from build123d import *

# Parameters (mm, degrees)
SKETCH_1_W          = 40
SKETCH_1_H          = 25
EXTRUDE_1_DEPTH     = 3
SKETCH_2_R          = 10.9
EXTRUDE_2_DEPTH     = 5
SKETCH_3_R          = 4
CUT_EXTRUDE_1_DEPTH = 25.904818811
CUT_EXTRUDE_2_DEPTH = 3.6
SKETCH_5_R          = 0.5
CUT_EXTRUDE_3_DEPTH = 4
FILLET_1_R          = 5
FILLET_2_R          = 5
FILLET_3_R          = 5
FILLET_4_R          = 5
SKETCH_6_R          = 7
SKETCH_6_R_2        = 3
EXTRUDE_3_DEPTH     = 10
SKETCH_7_R          = 4
SKETCH_7_R_2        = 2
EXTRUDE_4_DEPTH     = 3


with BuildPart() as part:
    # 草图1 → 凸台-拉伸1 (new body)
    with BuildSketch(Plane(origin=(0, 0, 0), x_dir=(1, 0, 0), z_dir=(0, 1, 0))):
        Rectangle(SKETCH_1_W, SKETCH_1_H)
    extrude(amount=EXTRUDE_1_DEPTH)

    # 草图2 → 凸台-拉伸2 (add)
    with BuildSketch(Plane(origin=(0, 3, 0), x_dir=(1, 0, 0), z_dir=(0, 1, 0))):
        with Locations(Location((0, 0, 0), (0, 0, 270))):
            Circle(SKETCH_2_R)
    extrude(amount=EXTRUDE_2_DEPTH)

    # 草图3 → 切除-拉伸1 (cut, through all)
    with BuildSketch(Plane.XZ):
        with Locations(Location((0, 0, 0), (0, 0, 270))):
            Circle(SKETCH_3_R)
    extrude(amount=-CUT_EXTRUDE_1_DEPTH, mode=Mode.SUBTRACT)

    # 草图4 → 切除-拉伸2 (cut)
    with BuildSketch(Plane(origin=(0, 8, 0), x_dir=(1, 0, 0), z_dir=(0, 1, 0))):
        Polygon((3.674809939, -1.579801226), (2.341337155, -12.320336373), (-2.341337155, -12.320336373), (-3.674809939, -1.579801226), align=None)
        Polygon((-3.674809939, 1.579801226), (-2.341337155, 12.320336373), (2.341337155, 12.320336373), (3.674809939, 1.579801226), align=None)
    extrude(amount=-CUT_EXTRUDE_2_DEPTH, mode=Mode.SUBTRACT)

    # 草图5 → 切除-拉伸3 (cut)
    with BuildSketch(Plane(origin=(0, 4.4, 0), x_dir=(1, 0, 0), z_dir=(0, 1, 0))):
        with Locations(Location((0, -6.5, 0), (0, 0, 270))):
            Circle(SKETCH_5_R)
        with Locations(Location((0, 6.5, 0), (0, 0, 270))):
            Circle(SKETCH_5_R)
    extrude(amount=-CUT_EXTRUDE_3_DEPTH, mode=Mode.SUBTRACT)

    # 圆角1
    fillet_1_edges = [part.edges().sort_by_distance(p)[0] for p in [
        (20, 1.5, 12.5),
    ]]
    fillet(fillet_1_edges, radius=FILLET_1_R)

    # 圆角2
    fillet_2_edges = [part.edges().sort_by_distance(p)[0] for p in [
        (-20, 1.5, 12.5),
    ]]
    fillet(fillet_2_edges, radius=FILLET_2_R)

    # 圆角3
    fillet_3_edges = [part.edges().sort_by_distance(p)[0] for p in [
        (-20, 1.5, -12.5),
    ]]
    fillet(fillet_3_edges, radius=FILLET_3_R)

    # 圆角4
    fillet_4_edges = [part.edges().sort_by_distance(p)[0] for p in [
        (20, 1.5, -12.5),
    ]]
    fillet(fillet_4_edges, radius=FILLET_4_R)

    # 草图6 → 凸台-拉伸3 (add)
    with BuildSketch(Plane(origin=(0, 0, 0), x_dir=(-1, 0, 0), z_dir=(0, -1, 0))):
        with Locations(Location((0, 0, 0), (0, 0, 270))):
            Circle(SKETCH_6_R)
        with Locations(Location((0, 0, 0), (0, 0, 90))):
            Circle(SKETCH_6_R_2, mode=Mode.SUBTRACT)
    extrude(amount=EXTRUDE_3_DEPTH)

    # 草图7 → 凸台-拉伸4 (add)
    with BuildSketch(Plane(origin=(0, 0, 0), x_dir=(1, 0, 0), z_dir=(0, 1, 0))):
        with Locations(Location((0, 0, 0), (0, 0, 156.73712516))):
            Circle(SKETCH_7_R)
        with Locations(Location((0, 0, 0), (0, 0, 270))):
            Circle(SKETCH_7_R_2, mode=Mode.SUBTRACT)
    extrude(amount=EXTRUDE_4_DEPTH)


solid = part.part
The listing builds one solid part. Answer for the finished solid, in the listing's coordinates (mm). A direction names the side the tool comes from. Give positions to 0.01 mm unless a question says otherwise; leave off trailing zeros. Loops run counter-clockwise (first coordinate to the right, second up) from the corner with the lowest first, then second, coordinate; pieces in that order, holes last.
Item 1: Each of these flat-tipped pins is pushed along its axis until it touches: pin 1 Ø0.8 at (x, z) = (0, 6.5) entering from +Y; pin 2 Ø4 at (x, z) = (-1, 1) entering from +Y; pin 3 Ø1.5 at (x, z) = (7, -8) entering from -Y. Where does it stop, or does it pass through?
Derived:
pin 1: stops at y = 0.4
pin 2: stops at y = 3
pin 3: stops at y = 0
Item 2: A cutting plane is placed at D-D (z = 9.25). Give the vertices of the cut face in (x, y), then the cut area to 3 significant figures.
Derived:
outline: (-19.68, 0) - (19.68, 0) - (19.68, 3) - (5.77, 3) - (5.77, 8) - (2.72, 8) - (2.72, 4.4) - (-2.72, 4.4) - (-2.72, 8) - (-5.77, 8) - (-5.77, 3) - (-19.68, 3) - close
area: 156 mm2
Item 3: A cutting plane is placed at C-C (y = 2). Give the vertices of the cut face in (x, z).
Derived:
outline: (-20, -7.5) arc R5 ccw to (-15, -12.5) - (15, -12.5) arc R5 ccw to (20, -7.5) - (20, 7.5) arc R5 ccw to (15, 12.5) - (-15, 12.5) arc R5 ccw to (-20, 7.5) - close; hole circle Ø4 at (0, 0); hole circle Ø1 at (0, -6.5); hole circle Ø1 at (0, 6.5)
Item 4: A cutting plane is placed at A-A (z = 0). Give the vertices of the cut face in (x, y).
Derived:
outline: (-20, 0) - (-7, 0) - (-7, -10) - (-3, -10) - (-3, 0) - (-2, 0) - (-2, 3) - (-4, 3) - (-4, 8) - (-10.9, 8) - (-10.9, 3) - (-20, 3) - close; (2, 0) - (3, 0) - (3, -10) - (7, -10) - (7, 0) - (20, 0) - (20, 3) - (10.9, 3) - (10.9, 8) - (4, 8) - (4, 3) - (2, 3) - close
Item 5: Determine the mould class of faces 1 (the flat face through (20, 1, 0)), 2 (the flat face through (3.123, 6.225, 6.025)), 3 (the flat face through (-5, 0, -6)) for opening direction X: +X half, -X half, draft (parallel to the pull), parting line (faces both ways), or undercut.
Derived:
face 1: +X half
face 2: undercut
face 3: draft
Item 6: Find the intervals of material crossed by line 1 along X through (y, z) = (-4.75, 0); line 2 along Y through (x, z) = (-2.5, 10.5); line 3 along X through (y, z) = (6.05, 0), in increasing order.
Derived:
line 1: x = -7 to -3, 3 to 7
line 2: y = 0 to 4.4
line 3: x = -10.9 to -4, 4 to 10.9
Item 7: A tool of negligible diameter and unlimited length cuts with its end or side. For faces 4 (the cylindrical face through (6.834, -4.93, -1.517)), 5 (the flat face through (7, 8, 0)), 6 (the cylindrical face through (3.27, 5.46, 10.4)), from which of +Z, -Z, +X, -X, +Y, -Y can it reach the whole face along a straight path? Write none if from no direction.
Derived:
face 4: -Y
face 5: +Z, -Z, +X, -X, +Y
face 6: +Y
